Here's how the part is built. I have some questions about the finished solid (model axes, mm). A direction names the side the tool comes from. Round coordinates to 2 decimals unless told otherwise and drop trailing zeros. Write each loop counter-clockwise with the first axis right and the second up, starting at its lowest first coordinate (ties: lowest second). Pieces come first, ordered by that corner, then holes. Notation, with made-up numbers: (-33.75, 88.25) - (-13.75, 88.25) arc R22 cw to (-13.75, 111.25) - close; hole circle Ø4 at (80, 6.5). An arc over 180 degrees is marked (long way). Write item = value, one per line. Start each with the question number.
Item 1: Thinking about a two-plate mould opening in X: for faces 3 (the face through (-63.5, 23, -44)), 4 (the face through (-1, 1.5, -44)), 5 (the face through (1, 0, -44)), which applies, pulls with the +X half, pulls with the -X half, needs draft (parallel to the pull), parting line crosses it, or undercut?
Item 2: If we section it at B-B (z = -52): Please give me the cut outline in (x, y), and give its area (3 significant figures).
Item 3: If we section it at C-C (x = -20): Please give me the cut outline in (y, z), and give its area (4 significant figures).
Item 4: If we section it at A-A (y = 23.5): Please give me the cut outline in (x, z), and give its area (3 significant figures).
Item 5: For P1, Ø1.5, axis at x = -31.5, z = -67, coming from the +Y side; P2, Ø2, axis at x = -40, z = -200, coming from the +Y side, each with a flat end and sliding along its axis, tell me the tip position at first contact or that it passes through.
Item 6: If I drill on line 1 along X through (y, z) = (1.15, -200); line 2 along X through (y, z) = (0.9, -200); line 3 along X through (y, z) = (28, -111), over which ranges is the centre line in solid material (lowest first)? Write a range as [from, to].
Item 7: Which directions (+Z, -Z, +X, -X, +Y, -Y) give clear straight access to the entire face, cutting with the end or side of a thin tool? Please do faces 1 (the face through (0, 1, -208)), 2 (the face through (62, 23, -44)).
```python
from build123d import *

# Parameters (mm, degrees)
SM_TRAY_DEPTH       = 333
SK_FACEHOLES_R      = 1.7
CUT_FACEHOLES_DEPTH = 1.5


# Sheet-metal steps are written as plain solids
with BuildPart() as part:
    # SK_Tray → SM_Tray (new body)
    with BuildSketch(Plane.XY.offset(-208)):
        with BuildLine():
            Line((-62, 43.5), (-62, 3))
            ThreePointArc((-62, 3), (-61.560660172, 1.939339828), (-60.5, 1.5))
            Line((-60.5, 1.5), (60.5, 1.5))
            ThreePointArc((60.5, 1.5), (61.560660172, 1.939339828), (62, 3))
            Line((62, 3), (62, 43.5))
            Line((62, 43.5), (63.5, 43.5))
            Line((63.5, 43.5), (63.5, 3))
            ThreePointArc((63.5, 3), (62.621320344, 0.878679656), (60.5, 0))
            Line((60.5, 0), (-60.5, 0))
            ThreePointArc((-60.5, 0), (-62.621320344, 0.878679656), (-63.5, 3))
            Line((-63.5, 3), (-63.5, 43.5))
            Line((-63.5, 43.5), (-62, 43.5))
        make_face()
    extrude(amount=SM_TRAY_DEPTH)

    # SK_FaceHoles → CUT_FaceHoles (cut)
    with BuildSketch(Plane(origin=(0, 0, 0), x_dir=(1, 0, 0), z_dir=(0, 1, 0))):
        with Locations(Location((40, 200, 0), (0, 0, 270))):
            Circle(SK_FACEHOLES_R)
        with Locations(Location((-40, 200, 0), (0, 0, 270))):
            Circle(SK_FACEHOLES_R)
    extrude(amount=CUT_FACEHOLES_DEPTH, mode=Mode.SUBTRACT)


solid = part.part
```
Reply:
q1.face_3 = pulls with the -X half
q1.face_4 = undercut
q1.face_5 = needs draft
q2.outline = (-63.5, 3) arc R3 ccw to (-60.5, 0) - (60.5, 0) arc R3 ccw to (63.5, 3) - (63.5, 43.5) - (62, 43.5) - (62, 3) arc R1.5 cw to (60.5, 1.5) - (-60.5, 1.5) arc R1.5 cw to (-62, 3) - (-62, 43.5) - (-63.5, 43.5) - close
q2.area = 314 mm2
q3.outline = (0, -208) - (1.5, -208) - (1.5, 125) - (0, 125) - close
q3.area = 499.5 mm2
q4.outline = (-63.5, -208) - (-62, -208) - (-62, 125) - (-63.5, 125) - close; (62, -208) - (63.5, -208) - (63.5, 125) - (62, 125) - close
q4.area = 999 mm2
q5.P1 = 1.5
q5.P2 = through
q6.line_1 = [-62.86, -41.7], [-38.3, 38.3], [41.7, 62.86]
q6.line_2 = [-62.64, -41.7], [-38.3, 38.3], [41.7, 62.64]
q6.line_3 = [-63.5, -62], [62, 63.5]
q7.face_1 = -Z, +X, -X, +Y, -Y
q7.face_2 = +Z, -Z, +Y
